The listing builds one solid part. Answer for the finished solid, in the listing's coordinates (mm). A direction names the side the tool comes from. Coordinates: 2 decimals unless noted, no trailing zeros. Order: outer loops, then holes, each group sorted by start corner. A loop starts at its lowest first (then second) coordinate and runs counter-clockwise, first axis right, second up. Notation, with made-up numbers: (-27, 8.25) -> (6, 8.25) arc R16 ccw to (6, 38.25) -> close; hole circle Ø5 at (-30.75, 8.25). An arc over 180 degrees is marked (long way). Return JSON: item names as keys, results as strings.
from build123d import *

# Parameters (mm, degrees)
SKETCH1_W                      = 400
SKETCH1_H                      = 90
BASE_FLANGE1_DEPTH             = 3
EDGE_FLANGE1_STRIP_W           = 18
EDGE_FLANGE1_STRIP_H           = 3
EDGE_FLANGE1_STRIP_CUT_DEPTH   = 90
EDGE_FLANGE1_STRIP_2_W         = 18
EDGE_FLANGE1_STRIP_2_H         = 3
EDGE_FLANGE1_STRIP_CUT_2_DEPTH = 90
EDGE_FLANGE1_DEPTH             = 90
EDGE_FLANGE1_BEND_DEPTH        = 90
SKETCH12_R                     = 2.5
CUT_EXTRUDE1_DEPTH             = 412.096095822


# Sheet-metal steps are written as plain solids
with BuildPart() as part:
    # Sketch1 → Base-Flange1 (new body)
    with BuildSketch(Plane(origin=(0, 0, 0), x_dir=(1, 0, 0), z_dir=(0, 1, 0))):
        with Locations((0, 45)):
            Rectangle(SKETCH1_W, SKETCH1_H)
    extrude(amount=-BASE_FLANGE1_DEPTH)

    # Edge-Flange1 strip (across the edge) → Edge-Flange1 strip cut (cut)
    with BuildSketch(Plane(origin=(-200, -3, 0), x_dir=(1, 0, 0), z_dir=(0, 0, -1))):
        with Locations((-3, -1.5)):
            Rectangle(EDGE_FLANGE1_STRIP_W, EDGE_FLANGE1_STRIP_H)
    extrude(amount=EDGE_FLANGE1_STRIP_CUT_DEPTH, mode=Mode.SUBTRACT)

    # Edge-Flange1 strip 2 (across the edge) → Edge-Flange1 strip cut 2 (cut)
    with BuildSketch(Plane(origin=(200, -3, -90), x_dir=(-1, 0, 0), z_dir=(0, 0, 1))):
        with Locations((-3, -1.5)):
            Rectangle(EDGE_FLANGE1_STRIP_2_W, EDGE_FLANGE1_STRIP_2_H)
    extrude(amount=EDGE_FLANGE1_STRIP_CUT_2_DEPTH, mode=Mode.SUBTRACT)

    # Edge-Flange1 section (across the edge) → Edge-Flange1 (add)
    with BuildSketch(Plane(origin=(-200, -3, 0), x_dir=(1, 0, 0), z_dir=(0, 0, -1))):
        with BuildLine():
            Line((0, 3), (0, 27))
            Line((0, 27), (3, 27))
            Line((3, 27), (3, 3))
            ThreePointArc((3, 3), (3.878679656, 0.878679656), (6, 0))
            Line((6, 0), (6, -3))
            ThreePointArc((6, -3), (1.757359313, -1.242640687), (0, 3))
        make_face()
    extrude(amount=EDGE_FLANGE1_DEPTH)

    # Edge-Flange1 section 2 (across the edge) → Edge-Flange1 bend (add)
    with BuildSketch(Plane(origin=(200, -3, -90), x_dir=(-1, 0, 0), z_dir=(0, 0, 1))):
        with BuildLine():
            Line((0, 3), (0, 27))
            Line((0, 27), (3, 27))
            Line((3, 27), (3, 3))
            ThreePointArc((3, 3), (3.878679656, 0.878679656), (6, 0))
            Line((6, 0), (6, -3))
            ThreePointArc((6, -3), (1.757359313, -1.242640687), (0, 3))
        make_face()
    extrude(amount=EDGE_FLANGE1_BEND_DEPTH)

    # Sketch12 → Cut-Extrude1 (cut, through all)
    with BuildSketch(Plane(origin=(200, 0, 0), x_dir=(0, 0, -1), z_dir=(1, 0, 0))):
        with Locations(Location((62.5, -18, 0), (0, 0, 90))):
            Circle(SKETCH12_R)
        with Locations(Location((27.5, -18, 0), (0, 0, 270))):
            Circle(SKETCH12_R)
    extrude(amount=-CUT_EXTRUDE1_DEPTH, mode=Mode.SUBTRACT)


solid = part.part
1. The part is cut by section B-B on x = 17.5. Give the vertices of the cut face in (y, z), and give its area (3 significant figures).
Answer block:
{"outline": "(-3, -90) -> (0, -90) -> (0, 0) -> (-3, 0) -> close", "area": "270 mm2"}
2. The part is cut by section A-A on z = -47. Give the vertices of the cut face in (x, y), and give its area (3 significant figures).
Answer block:
{"outline": "(-200, -30) -> (-197, -30) -> (-197, -6) arc R3 cw to (-194, -3) -> (194, -3) arc R3 cw to (197, -6) -> (197, -30) -> (200, -30) -> (200, -6) arc R6 ccw to (194, 0) -> (-194, 0) arc R6 ccw to (-200, -6) -> close", "area": "1,350 mm2"}
3. Consider line 1 (Z direction, x = -198.6, y = -18); line 2 (X direction, y = -21, z = -9); line 3 (Y direction, x = -103, z = -53). Determine where each line is inside the solid, lowest interval first. Write a range as from..to.
Answer block:
{"line 1": "z = -90..-65, -60..-30, -25..0", "line 2": "x = -200..-197, 197..200", "line 3": "y = -3..0"}
4. For faces 1 (the face through (197, -18, -46)), 2 (the face through (-200, -18, -44)), determine the directions among +Z, -Z, +X, -X, +Y, -Y from which every point of the face is accessible in a straight line to the end or side of a thin tool.
Answer block:
{"face 1": "+Z, -Z, -Y", "face 2": "+Z, -Z, -X, +Y, -Y"}
5. Determine the mould class of faces 3 (the face through (-1, -2, -90)), 4 (the face through (-197, -18, -44)), 5 (the face through (200, -18, -46)), 6 (the face through (-3, -3, -46)) for opening direction X: pulls with the +X half, pulls with the -X half, needs draft (parallel to the pull), parting line crosses it, or undercut.
Answer block:
{"face 3": "needs draft", "face 4": "undercut", "face 5": "pulls with the +X half", "face 6": "undercut"}
6. Each of these flat-tipped pins is pushed along its axis until it touches: pin 1 Ø8 at (y, z) = (-18, -27.5) entering from +X; pin 2 Ø3 at (x, z) = (-59.5, -19.5) entering from -Y. Where does it stop, or does it pass through?
Answer block:
{"pin 1": "stops at x = 200", "pin 2": "stops at y = -3"}
